Design review of the part built by this model. Coordinates are the model's own, in mm. A direction names the side the tool comes from. Give positions to 0.01 mm unless a question says otherwise; leave off trailing zeros. Write each loop counter-clockwise with the first axis right and the second up, starting at its lowest first coordinate (ties: lowest second). Pieces come first, ordered by that corner, then holes.
```python
from build123d import *

# Parameters (mm, degrees)
SKETCH1_W           = 120
SKETCH1_H           = 80
SKETCH1_W_2         = 115
SKETCH1_H_2         = 76.666666666
BOSS_EXTRUDE1_DEPTH = 20
SKETCH1_3_W         = 115
SKETCH1_3_H         = 76.666666666
BOSS_EXTRUDE2_DEPTH = 2.5
SKETCH2_R           = 13.5
CUT_EXTRUDE1_DEPTH  = 129.062484749


with BuildPart() as part:
    # Sketch1 → Boss-Extrude1 (new body)
    with BuildSketch(Plane(origin=(0, 0, 0), x_dir=(1, 0, 0), z_dir=(0, 1, 0))):
        Rectangle(SKETCH1_W, SKETCH1_H)
        Rectangle(SKETCH1_W_2, SKETCH1_H_2, mode=Mode.SUBTRACT)
    extrude(amount=BOSS_EXTRUDE1_DEPTH)

    # Sketch1<3> → Boss-Extrude2 (add)
    with BuildSketch(Plane(origin=(0, 0, 0), x_dir=(1, 0, 0), z_dir=(0, 1, 0))):
        Rectangle(SKETCH1_3_W, SKETCH1_3_H)
    extrude(amount=BOSS_EXTRUDE2_DEPTH)

    # Sketch2 → Cut-Extrude1 (cut, through all)
    with BuildSketch(Plane.ZY.offset(60)):
        with Locations((0, 16)):
            Circle(SKETCH2_R)
    extrude(amount=-CUT_EXTRUDE1_DEPTH, mode=Mode.SUBTRACT)


solid = part.part
```
(1) Mouldability with a two-part tool opening along Y and no side actions: class faces 1 (the face through (-18, 20, -39)), 2 (the face through (-1, 10, -40)), 3 (the face through (58.732, 2.505, -0.354)) as pulls with the +Y half, pulls with the -Y half, needs draft (parallel to the pull), parting line crosses it, or undercut.
Resolved:
face 1: pulls with the +Y half
face 2: needs draft
face 3: undercut
(2) To check wall thickness, follow L1, parallel to Z at x = 46, y = 16.5; L2, parallel to X at y = 9.75, z = 12; L3, parallel to Z at x = 58.5, y = 16. State the ranges of each line that lie inside material, in increasing order.
Resolved:
L1: z = -40 to -38.33, 38.33 to 40
L2: x = -60 to -57.5, 57.5 to 60
L3: z = -40 to -13.5, 13.5 to 40
(3) Consider section D-D, the plane y = 3.75. Give the boundary of the cut face in (x, z).
Resolved:
outline: (-60, -40) - (60, -40) - (60, -5.67) - (57.5, -5.67) - (57.5, -38.33) - (-57.5, -38.33) - (-57.5, -5.67) - (-60, -5.67) - close; (-60, 5.67) - (-57.5, 5.67) - (-57.5, 38.33) - (57.5, 38.33) - (57.5, 5.67) - (60, 5.67) - (60, 40) - (-60, 40) - close
(4) Clearance check with a flat-ended pin moving along its axis: P1, Ø10, axis at x = -38.5, z = -28, coming from the +Y side. State where the tip first meets the part, or that it passes through.
Resolved:
P1: stops at y = 2.5
(5) Consider section A-A, the plane y = 16. Give the boundary of the cut face in (x, z).
Resolved:
outline: (-60, -40) - (60, -40) - (60, -13.5) - (57.5, -13.5) - (57.5, -38.33) - (-57.5, -38.33) - (-57.5, -13.5) - (-60, -13.5) - close; (-60, 13.5) - (-57.5, 13.5) - (-57.5, 38.33) - (57.5, 38.33) - (57.5, 13.5) - (60, 13.5) - (60, 40) - (-60, 40) - close
(6) Consider section B-B, the plane z = -26. Give the boundary of the cut face in (x, y).
Resolved:
outline: (-60, 0) - (60, 0) - (60, 20) - (57.5, 20) - (57.5, 2.5) - (-57.5, 2.5) - (-57.5, 20) - (-60, 20) - close
(7) Consider section C-C, the plane x = 10. Give the boundary of the cut face in (y, z), then the cut area to 3 significant figures.
Resolved:
outline: (0, -40) - (20, -40) - (20, -38.33) - (2.5, -38.33) - (2.5, 38.33) - (20, 38.33) - (20, 40) - (0, 40) - close
area: 258 mm2
(8) Tool access review of faces 4 (the face through (-57.5, 11, -23)), 5 (the face through (-18, 20, 39)): name each direction out of +Z, -Z, +X, -X, +Y, -Y from which nothing blocks a thin tool from reaching the whole face with its end or side.
Resolved:
face 4: +Y
face 5: +Z, -Z, +X, -X, +Y
